from build123d import *

# Parameters (mm, degrees)
F0_W     = 49.8126782477
F0_H     = 66.5889680386
F1_DEPTH = 19.812
F2_T     = -2.54
F3_R     = 15.24


with BuildPart() as f1:
    # F0 (on Top) → F1 (new body)
    with BuildSketch(Plane.XY):
        with Locations((-5.807178095, 4.1295476258)):
            Rectangle(F0_W, F0_H)
    extrude(amount=-F1_DEPTH)

    # F2
    f2_openings = [f1.faces().sort_by_distance(p)[0] for p in [
        (-5.807178, 4.129548, 0),
    ]]
    offset(amount=F2_T, openings=f2_openings)

    # F3
    f3_edges = [f1.edges().sort_by_distance(p)[0] for p in [
        (16.559161, 4.129548, -17.272),
        (-5.807178, -26.624936, -17.272),
        (-5.807178, 34.884032, -17.272),
        (-28.173517, 4.129548, -17.272),
    ]]
    fillet(f3_edges, radius=F3_R)


solid = f1.part
Read the model definition and answer for the solid it produces. Units are mm, in the model's axes. A direction names the side the tool comes from. Coordinates: 2 decimals unless noted, no trailing zeros. Order: outer loops, then holes, each group sorted by start corner. A loop starts at its lowest first (then second) coordinate and runs counter-clockwise, first axis right, second up. Notation, with made-up numbers: (25.5, -35) -> (29.5, -35) arc R23 cw to (29.5, -27) -> close; hole circle Ø4 at (22, -37.5). An arc over 180 degrees is marked (long way). Answer as a JSON object with one key per item and string values.
1) Each of these flat-tipped pins is pushed along its axis until it touches: pin 1 (6 mm diameter, centred on x = -18, y = -11, fed in from +Z); pin 2 (8 mm diameter, centred on x = 14, y = 26.5, fed in from +Z); pin 3 (4.5 mm diameter, centred on x = -5.5, y = 4.5, fed in from +Z). Where does it stop, or does it pass through?
Model answer:
{"pin 1": "stops at z = -14.96", "pin 2": "stops at z = 0", "pin 3": "stops at z = -17.27"}
2) The mould has two halves that part along X. Classify faces 3 (the face through (-30, 4, 0)), 4 (the face through (-6, 34.884, -1)), 5 (the face through (-30.714, 4, -10)): released by +X, released by -X, zero draft, split by the parting line, or undercut.
Model answer:
{"face 3": "zero draft", "face 4": "undercut", "face 5": "released by -X"}
3) Consider line 1 along Y through (x, z) = (-13, -1); line 2 along X through (y, z) = (24, -1.75); line 3 along Y through (x, z) = (0.5, -10.25). Determine where each line is inside the solid, lowest interval first. Write a range as from..to.
Model answer:
{"line 1": "y = -29.16..-26.62, 34.88..37.42", "line 2": "x = -30.71..-28.17, 16.56..19.1", "line 3": "y = -29.16..-24.22, 32.48..37.42"}
4) A tool of negligible diameter and unlimited length cuts with its end or side. For faces 1 (the face through (-6, 37.424, -10)), 2 (the face through (-6.12, 32.22, -10.64)), from which of +Z, -Z, +X, -X, +Y, -Y can it reach the whole face along a straight path? Write none if from no direction.
Model answer:
{"face 1": "+Z, -Z, +X, -X, +Y", "face 2": "+Z"}
5) A cutting plane is placed at A-A, the plane z = -12.75. Determine the outline of the cut face in (x, y).
Model answer:
{"outline": "(-30.71, -29.16) -> (19.1, -29.16) -> (19.1, 37.42) -> (-30.71, 37.42) -> close; hole (-23.77, -22.22) -> (12.15, -22.22) -> (12.15, 30.48) -> (-23.77, 30.48) -> close"}
6) A cutting plane is placed at B-B, the plane y = 4.5. Determine the outline of the cut face in (x, z), plus the area to 3 significant figures.
Model answer:
{"outline": "(-30.71, -19.81) -> (19.1, -19.81) -> (19.1, 0) -> (16.56, 0) -> (16.56, -2.03) arc R15.24 cw to (1.32, -17.27) -> (-12.93, -17.27) arc R15.24 cw to (-28.17, -2.03) -> (-28.17, 0) -> (-30.71, 0) -> close", "area": "314 mm²"}
7) A cutting plane is placed at D-D, the plane z = -5.5. Determine the outline of the cut face in (x, y).
Model answer:
{"outline": "(-30.71, -29.16) -> (19.1, -29.16) -> (19.1, 37.42) -> (-30.71, 37.42) -> close; hole (-27.77, -26.23) -> (16.16, -26.23) -> (16.16, 34.48) -> (-27.77, 34.48) -> close"}
8) A cutting plane is placed at C-C, the plane x = -1. Determine the outline of the cut face in (y, z).
Model answer:
{"outline": "(-29.16, -19.81) -> (37.42, -19.81) -> (37.42, 0) -> (34.88, 0) -> (34.88, -2.03) arc R15.24 cw to (19.64, -17.27) -> (-11.38, -17.27) arc R15.24 cw to (-26.62, -2.03) -> (-26.62, 0) -> (-29.16, 0) -> close"}
